Part model, mm, in its own coordinate system. Face numbers are marked on the shaded views. A direction names the side the tool comes from. Round coordinates to 2 decimals unless told otherwise and drop trailing zeros. Loops run counter-clockwise (first coordinate to the right, second up) from the corner with the lowest first, then second, coordinate; pieces in that order, holes last. Notation, with made-up numbers: (-13, 83.25) -> (20, 83.25) arc R22 ccw to (20, 98.25) -> close; hole circle Ø3 at (9, 71.25). An arc over 180 degrees is marked (long way). Answer as CSV lines item,"result".
from build123d import *

# Parameters (mm, degrees)
PAD_DEPTH       = 3
SKETCH001_W     = 32
SKETCH001_H     = 60
PAD001_DEPTH    = 32
SKETCH002_W     = 22
SKETCH002_H     = 54
POCKET_DEPTH    = 32
SKETCH003_W     = 38
SKETCH003_H     = 10
PAD002_DEPTH    = 15
POCKET001_DEPTH = 32
SKETCH005_W     = 32
SKETCH005_H     = 31
PAD003_DEPTH    = 32
SKETCH006_W     = 13.2
SKETCH006_H     = 13.2
POCKET002_DEPTH = 32
SKETCH007_W     = 1.848
SKETCH007_H     = 4.499
POCKET003_DEPTH = 10.55


with BuildPart() as part:
    # Sketch → Pad (new body)
    with BuildSketch(Plane.XY):
        Polygon((-48.115829, 15.5), (21.884171, 15.5), (21.884171, 30), (53.884171, 30), (53.884171, -30), (21.884171, -30), (21.884171, -15.5), (-48.115829, -15.5), align=None)
    extrude(amount=PAD_DEPTH)

    # Sketch001 (on Face10 of Pad) → Pad001 (join)
    with BuildSketch(Plane.XY.offset(3)):
        with Locations((37.884171, 0)):
            Rectangle(SKETCH001_W, SKETCH001_H)
    extrude(amount=PAD001_DEPTH)

    # Sketch002 (on Face14 of Pad001) → Pocket (cut)
    with BuildSketch(Plane.XY.offset(35)):
        with Locations((42.884171, 0)):
            Rectangle(SKETCH002_W, SKETCH002_H)
    extrude(amount=-POCKET_DEPTH, mode=Mode.SUBTRACT)

    # Sketch003 (on Face5 of Pocket) → Pad002 (join)
    with BuildSketch(Plane.XY.offset(3)):
        with Locations((2.884171, 0)):
            Rectangle(SKETCH003_W, SKETCH003_H)
    extrude(amount=PAD002_DEPTH)

    # Sketch004 (on Face17 of Pad002) → Pocket001 (cut)
    with BuildSketch(Plane.XY.offset(35)):
        Polygon((31.884171, 10), (31.884171, -10), (26.884171, -10), (26.884171, -2.5), (11.884171, -2.5), (11.884171, 2.5), (26.884171, 2.5), (26.884171, 10), align=None)
    extrude(amount=-POCKET001_DEPTH, mode=Mode.SUBTRACT)

    # Sketch005 (on Face5 of Pocket001) → Pad003 (join)
    with BuildSketch(Plane.XY.offset(3)):
        with Locations((-32.115829, 0)):
            Rectangle(SKETCH005_W, SKETCH005_H)
    extrude(amount=PAD003_DEPTH)

    # Sketch006 (on Face15 of Pad003) → Pocket002 (cut)
    with BuildSketch(Plane.XY.offset(35)):
        with Locations((-32.115829, 0)):
            Rectangle(SKETCH006_W, SKETCH006_H)
    extrude(amount=-POCKET002_DEPTH, mode=Mode.SUBTRACT)

    # Sketch007 (on Face21 of Pocket002) → Pocket003 (cut)
    with BuildSketch(Plane.XY.offset(18)):
        with Locations((3.484171, 0)):
            Rectangle(SKETCH007_W, SKETCH007_H)
    extrude(amount=-POCKET003_DEPTH, mode=Mode.SUBTRACT)


solid = part.part
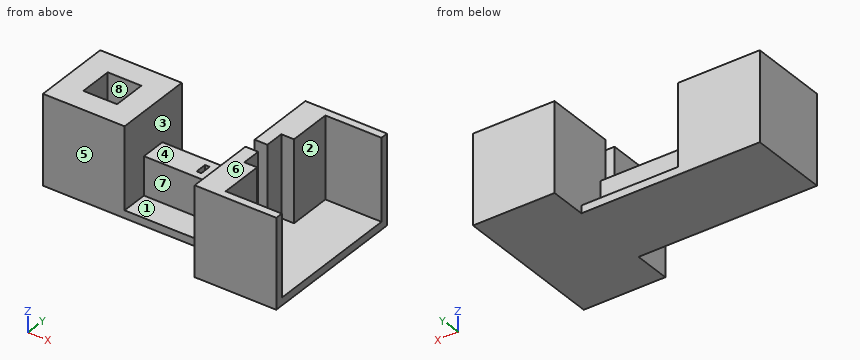
Q1. Saw through at B-B, the plane x = 8. Write the cut outline in (y, z), then the cut area to 3 significant figures.
Geometry results:
outline,"(-15.5, 0) -> (15.5, 0) -> (15.5, 3) -> (5, 3) -> (5, 18) -> (-5, 18) -> (-5, 3) -> (-15.5, 3) -> close"
area,"243 mm2"
Q2. Two-plate mould, pull along Y, no slides. Class the marked faces 6, 7 and 8: pulls with the +Y half, pulls with the -Y half, needs draft (parallel to the pull), parting line crosses it, or undercut.
Geometry results:
face 6,"needs draft"
face 7,"pulls with the -Y half"
face 8,"undercut"
Q3. Drop flat-ended pins along their axis: P1, Ø9.5, axis at y = -3, z = 26.5, coming from the +X side; P2, Ø1.5, axis at x = 3, z = 13.5, coming from the +Y side; P3, Ø4.5, axis at x = 15.5, z = 20.5, coming from the -Y side; P4, Ø4, axis at y = 15, z = 25.5, coming from the +X side. Give the stop position or say it passes through.
Geometry results:
P1,"x = 26.88"
P2,"y = 5"
P3,"through"
P4,"x = 31.88"
Q4. Saw through at C-C, the plane z = 16.5. Give the number of separate pieces and of enclosed holes in the cut face, then the cut area to 3 significant figures.
Geometry results:
separate pieces,"1"
enclosed holes,"2"
area,"1,750 mm2"
Q5. Drill centre lines: line 1 along Y through (x, z) = (49.5, 16); line 2 along X through (y, z) = (9.5, 26); line 3 along Y through (x, z) = (25.5, 4). Where is each one in solid material? Low to high.
Geometry results:
line 1,"-30 to -27, 27 to 30"
line 2,"-48.12 to -16.12, 21.88 to 26.88"
line 3,"-30 to -2.5, 2.5 to 30"
Q6. Saw through at D-D, the plane y = 4. Write the cut outline in (x, z), then the cut area to 3 significant figures.
Geometry results:
outline,"(-48.12, 0) -> (53.88, 0) -> (53.88, 3) -> (26.88, 3) -> (26.88, 35) -> (21.88, 35) -> (21.88, 18) -> (-16.12, 18) -> (-16.12, 35) -> (-25.52, 35) -> (-25.52, 3) -> (-38.72, 3) -> (-38.72, 35) -> (-48.12, 35) -> close"
area,"1,640 mm2"
Q7. Saw through at A-A, the plane z = 21.5. Write the cut outline in (x, y), then the cut area to 3 significant figures.
Geometry results:
outline,"(-48.12, -15.5) -> (-16.12, -15.5) -> (-16.12, 15.5) -> (-48.12, 15.5) -> close; (21.88, -30) -> (53.88, -30) -> (53.88, -27) -> (31.88, -27) -> (31.88, -10) -> (26.88, -10) -> (26.88, -2.5) -> (21.88, -2.5) -> close; (21.88, 2.5) -> (26.88, 2.5) -> (26.88, 10) -> (31.88, 10) -> (31.88, 27) -> (53.88, 27) -> (53.88, 30) -> (21.88, 30) -> close; hole (-38.72, -6.6) -> (-25.52, -6.6) -> (-25.52, 6.6) -> (-38.72, 6.6) -> close"
area,"1,420 mm2"
Q8. Which spindle directions (+Z, -Z, +X, -X, +Y, -Y) get a long thin tool onto all of the face, cutting with end or side? Do the marked faces 1, 2, 3, 4 and 5. Say none if no direction does.
Geometry results:
face 1,"+Z, -Y"
face 2,"+Z, +X"
face 3,"+Z"
face 4,"+Z, +Y, -Y"
face 5,"+Z, -Z, -X, -Y"
